The listing builds one solid part. Answer for the finished solid, in the listing's coordinates (mm). A direction names the side the tool comes from. Give positions to 0.01 mm unless a question says otherwise; leave off trailing zeros. Loops run counter-clockwise (first coordinate to the right, second up) from the corner with the lowest first, then second, coordinate; pieces in that order, holes last.
Item 1: A tool of negligible diameter and unlimited length cuts with its end or side. For faces 1 (the face through (20, 10, 1)), 2 (the face through (-24, 15, 1)), 3 (the face through (23, 25, 1)), 4 (the face through (-24, 25, 1)), 5 (the face through (-24, -25, 1)), from which of +Z, -Z, +X, -X, +Y, -Y can it reach the whole face along a straight path? Write none if from no direction.
Item 2: Section A-A, the plane x = -21 is taken. Give the vertices of the cut face in (y, z), and give its area (3 significant figures).
Item 3: Section C-C, the plane y = -28 is taken. Give the vertices of the cut face in (x, z).
Item 4: Consider line 1 along Y through (x, z) = (25.5, 0.7); line 2 along X through (y, z) = (-31, 2). Determine where each line is inside the solid, lowest interval first.
Item 5: Section B-B, the plane z = 1.2 is taken. Give the vertices of the cut face in (x, y).
Item 6: Each of these flat-tipped pins is pushed along its axis until it touches: pin 1 Ø0.9 at (x, z) = (-22.5, 1) entering from -Y; pin 2 Ø1.5 at (x, z) = (-22.5, 2) entering from +Y; pin 3 Ø0.9 at (y, z) = (11, 1.5) entering from -X. Where does it stop, or does it pass through?
Item 7: The mould has two halves that part along Y. Classify faces 6 (the face through (0, 35, 1)), 7 (the face through (20, 30, 1)), 8 (the face through (23, -15, 1)): pulls with the +Y half, pulls with the -Y half, needs draft (parallel to the pull), parting line crosses it, or undercut.
from build123d import *

# Parameters (mm, degrees)
ESBO_O1_W                = 7
ESBO_O1_H                = 10
RESSALTO_EXTRUS_O1_DEPTH = 3


with BuildPart() as part:
    # Esboço1 → Ressalto-extrusão1 (new body)
    with BuildSketch(Plane.XY):
        with Locations((-23.5, 0)):
            Rectangle(ESBO_O1_W, ESBO_O1_H)
        with Locations((-23.5, -20)):
            Rectangle(ESBO_O1_W, ESBO_O1_H)
        with Locations((23.5, 20)):
            Rectangle(ESBO_O1_W, ESBO_O1_H)
        with Locations((23.5, 0)):
            Rectangle(ESBO_O1_W, ESBO_O1_H)
        with Locations((23.5, -20)):
            Rectangle(ESBO_O1_W, ESBO_O1_H)
        Polygon((0, -35), (0, 35), (-20, 35), (-20, 25), (-20, 15), (-20, 5), (-20, -5), (-20, -15), (-20, -25), (-20, -35), align=None)
        Polygon((20, 35), (0, 35), (0, -35), (20, -35), (20, -25), (20, -15), (20, -5), (20, 5), (20, 15), (20, 25), align=None)
        with Locations((-23.5, 20)):
            Rectangle(ESBO_O1_W, ESBO_O1_H)
    extrude(amount=RESSALTO_EXTRUS_O1_DEPTH)


solid = part.part
Worked answers:
1. face 1: +Z, -Z, +X
1. face 2: +Z, -Z, -X
1. face 3: +Z, -Z, +X, +Y
1. face 4: +Z, -Z, -X, +Y
1. face 5: +Z, -Z, -X, -Y
2. outline: (-25, 0) - (-15, 0) - (-15, 3) - (-25, 3) - close; (-5, 0) - (5, 0) - (5, 3) - (-5, 3) - close; (15, 0) - (25, 0) - (25, 3) - (15, 3) - close
2. area: 90.0 mm2
3. outline: (-20, 0) - (20, 0) - (20, 3) - (-20, 3) - close
4. line 1: y = -25 to -15, -5 to 5, 15 to 25
4. line 2: x = -20 to 20
5. outline: (-27, -25) - (-20, -25) - (-20, -35) - (20, -35) - (20, -25) - (27, -25) - (27, -15) - (20, -15) - (20, -5) - (27, -5) - (27, 5) - (20, 5) - (20, 15) - (27, 15) - (27, 25) - (20, 25) - (20, 35) - (-20, 35) - (-20, 25) - (-27, 25) - (-27, 15) - (-20, 15) - (-20, 5) - (-27, 5) - (-27, -5) - (-20, -5) - (-20, -15) - (-27, -15) - close
6. pin 1: stops at y = -25
6. pin 2: stops at y = 25
6. pin 3: stops at x = -20
7. face 6: pulls with the +Y half
7. face 7: needs draft
7. face 8: undercut
